Geometry: final body of the model. Coordinates: model frame, mm. Face numbers are marked on the shaded views. A direction names the side the tool comes from. Give positions to 0.01 mm unless a question says otherwise; leave off trailing zeros. Write each loop counter-clockwise with the first axis right and the second up, starting at its lowest first coordinate (ties: lowest second). Pieces come first, ordered by that corner, then holes.
Q1. Section B-B (x = 132.5). Return the cut outline in (y, z), plus the area to 3 significant figures.
Q2. Line query: line 1 (Y direction, x = 152.5, z = 1105); line 2 (Z direction, x = 134.5, y = -183); line 3 (Z direction, x = 113, y = -221). Output: solid intervals per line, ascending.
Q3. Section A-A (z = 1002). Return the cut outline in (x, y), plus the area to 3 significant figures.
Q4. Pin query (flat end, axial travel): pin 1 Ø1 at (x, y) = (-33, -258) entering from -Z; pin 2 Ø10 at (x, y) = (-18.5, -221) entering from -Z; pin 3 Ø2 at (x, y) = (86, -214) entering from -Z. Return the tip coordinate at first contact, or that it passes through.
Q5. Section C-C (y = -253). Return the cut outline in (x, z), plus the area to 3 significant figures.
Q6. Reachability of the marked faces 5 and 6 from +Z, -Z, +X, -X, +Y, -Y: full face, straight path, thin tool, end or side. Return the list, or none.
Q7. Mould query, pull axis Z, two halves, no side actions, for the marked faces 1, 2, 3 and 4. Classes: +Z half, -Z half, draft (parallel to the pull), parting line (faces both ways), or undercut.
Autodesk Inventor part; units mm, degrees
ref_plane "YZ Plane" through (0, 0, 0) normal (1, 0, 0) x (0, 1, 0)
ref_plane "XZ Plane" through (0, 0, 0) normal (0, 1, 0) x (-1, 0, 0)
ref_plane "XY Plane" through (0, 0, 0) normal (0, 0, 1) x (1, 0, 0)
sketch "Skizze3" plane through (0, 0, 0) normal (1, 0, 0) x (0, 1, 0)
  line L0 (-97.3116, 946.0308) -> (-97.3116, 624.8101)
  arc A0 (-297.3116, 624.8101) -> (-97.3116, 624.8101) centre (-197.3116, 624.8101) ccw
  line L1 (-297.3116, 624.8101) -> (-297.3116, 1009.2763)
  line L2 (-97.3116, 946.0308) -> (-97.3116, 1267.2514)
  arc A1 (-97.3116, 1267.2514) -> (-297.3116, 1267.2514) centre (-197.3116, 1267.2514) ccw
  line L3 (-297.3116, 1267.2514) -> (-297.3116, 1009.2763)
  line L4 (-87.3116, 946.0308) -> (-87.3116, 624.8101)
  arc A2 (-307.3116, 624.8101) -> (-87.3116, 624.8101) centre (-197.3116, 624.8101) ccw
  line L5 (-307.3116, 624.8101) -> (-307.3116, 946.0308)
  line L6 (-87.3116, 946.0308) -> (-307.3116, 946.0308)
  line L7 (-307.3116, 1267.2514) -> (-307.3116, 946.0308)
  line L8 (-87.3116, 946.0308) -> (-87.3116, 1267.2514)
  arc A3 (-87.3116, 1267.2514) -> (-307.3116, 1267.2514) centre (-197.3116, 1267.2514) ccw
  point P0 (0, 0)
  dimension "d0" = 110
  dimension "d1" = 100
extrude "Extrusion1" add sketch "Skizze3" along normal mid plane 400 contours L6 L4 A2 L5 L1 A0 L0 | L2 A1 L3 L1 L6 L7 A3 L8
properties part number "Förderband"
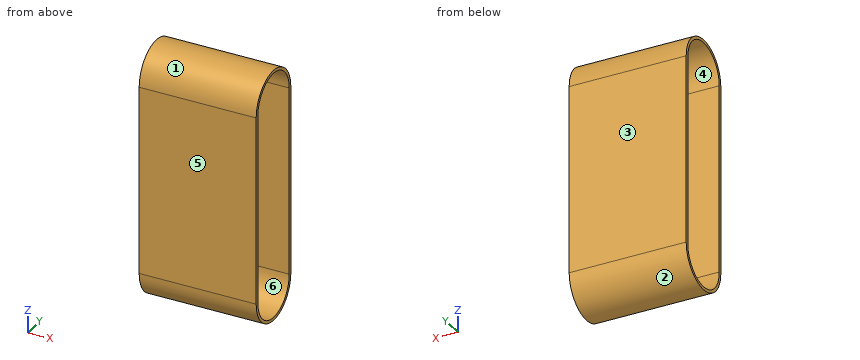
Computed:
1. outline: (-307.31, 624.81) arc R110 ccw to (-87.31, 624.81) - (-87.31, 1267.25) arc R110 ccw to (-307.31, 1267.25) - close; hole (-297.31, 624.81) arc R100 ccw to (-97.31, 624.81) - (-97.31, 1267.25) arc R100 ccw to (-297.31, 1267.25) - close
1. area: 19,400 mm2
2. line 1: y = -307.31 to -297.31, -97.31 to -87.31
2. line 2: z = 515.75 to 525.84, 1366.22 to 1376.32
2. line 3: z = 517.39 to 527.66, 1364.41 to 1374.67
3. outline: (-200, -307.31) - (200, -307.31) - (200, -297.31) - (-200, -297.31) - close; (-200, -97.31) - (200, -97.31) - (200, -87.31) - (-200, -87.31) - close
3. area: 8,000 mm2
4. pin 1: stops at z = 532.74
4. pin 2: stops at z = 516.41
4. pin 3: stops at z = 515.93
5. outline: (-200, 529.95) - (200, 529.95) - (200, 541.75) - (-200, 541.75) - close; (-200, 1350.31) - (200, 1350.31) - (200, 1362.11) - (-200, 1362.11) - close
5. area: 9,440 mm2
6. face 5: +Z, -Z, +X, -X, -Y
6. face 6: +X, -X
7. face 1: +Z half
7. face 2: -Z half
7. face 3: draft
7. face 4: undercut
